```python
from build123d import *

# Parameters (mm, degrees)
SKETCH1_W           = 863.6
SKETCH1_H           = 184.15
BOSS_EXTRUDE1_DEPTH = 38.1
SKETCH3_W           = 88.9
SKETCH3_H           = 40.5765
CUT_EXTRUDE1_DEPTH  = 39.1


with BuildPart() as part:
    # Sketch1 → Boss-Extrude1 (new body)
    with BuildSketch(Plane(origin=(0, 0, 0), x_dir=(1, 0, 0), z_dir=(0, 1, 0))):
        with Locations((431.8, 92.075)):
            Rectangle(SKETCH1_W, SKETCH1_H)
    extrude(amount=BOSS_EXTRUDE1_DEPTH)

    # Sketch3 → Cut-Extrude1 (cut, through all)
    with BuildSketch(Plane(origin=(0, 38.1, 0), x_dir=(1, 0, 0), z_dir=(0, 1, 0))):
        with Locations((44.45, 163.86175)):
            Rectangle(SKETCH3_W, SKETCH3_H)
        Polygon((863.6, 78.486), (774.7, 78.486), (774.7, 40.386), (679.45, 40.386), (679.45, 0), (863.6, 0), align=None)
    extrude(amount=-CUT_EXTRUDE1_DEPTH, mode=Mode.SUBTRACT)


solid = part.part
```
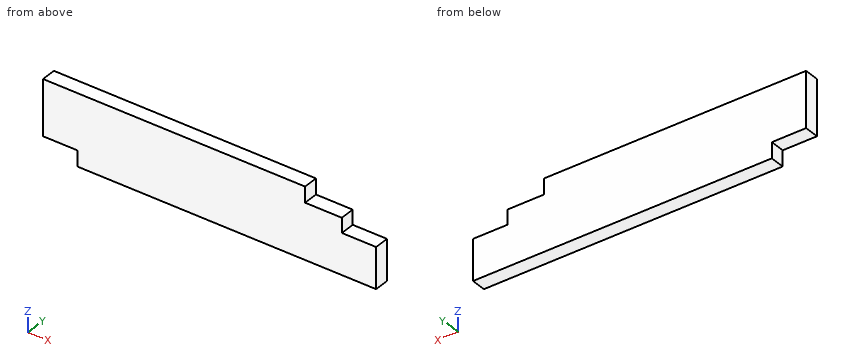
Geometry: final body of the model. Coordinates: model frame, mm. Round coordinates to 2 decimals unless told otherwise and drop trailing zeros. Write each loop counter-clockwise with the first axis right and the second up, starting at its lowest first coordinate (ties: lowest second). Pieces come first, ordered by that corner, then holes. Notation, with made-up numbers: (-38, -3.75) -> (-14, -3.75) arc R20 ccw to (-14, 24.25) -> close; hole circle Ø1 at (84.5, 71.5). An arc over 180 degrees is marked (long way). Return JSON: item names as keys, results as strings.
Q1. Ray query, line 1 (Z direction, x = 757, y = 28); line 2 (Z direction, x = 66, y = 27.5); line 3 (X direction, y = 5.5, z = -47). Return the intervals inside material, ascending.
From the geometry:
{"line 1": "-184.15 to -40.39", "line 2": "-143.57 to 0", "line 3": "0 to 774.7"}
Q2. Section C-C on x = 710.5. Return the cut outline in (y, z), and give its area (3 significant figures).
From the geometry:
{"outline": "(0, -184.15) -> (38.1, -184.15) -> (38.1, -40.39) -> (0, -40.39) -> close", "area": "5,480 mm2"}
Q3. Section B-B on z = -60. Return the cut outline in (x, y), and give its area (3 significant figures).
From the geometry:
{"outline": "(0, 0) -> (774.7, 0) -> (774.7, 38.1) -> (0, 38.1) -> close", "area": "29,500 mm2"}
Q4. First-contact query: pin 1 Ø11.5 at (y, z) = (10.5, -167) entering from -X; pin 2 Ø19 at (x, y) = (42, 14) entering from -Z; pin 3 Ø2 at (x, y) = (775.5, 19.5) entering from +Z. Flat tips, straight axial feed; report the tip coordinate or a pass-through.
From the geometry:
{"pin 1": "x = 88.9", "pin 2": "z = -143.57", "pin 3": "z = -40.39"}
Q5. Section A-A on y = 24.5. Return the cut outline in (x, z).
From the geometry:
{"outline": "(0, -143.57) -> (88.9, -143.57) -> (88.9, -184.15) -> (863.6, -184.15) -> (863.6, -78.49) -> (774.7, -78.49) -> (774.7, -40.39) -> (679.45, -40.39) -> (679.45, 0) -> (0, 0) -> close"}
